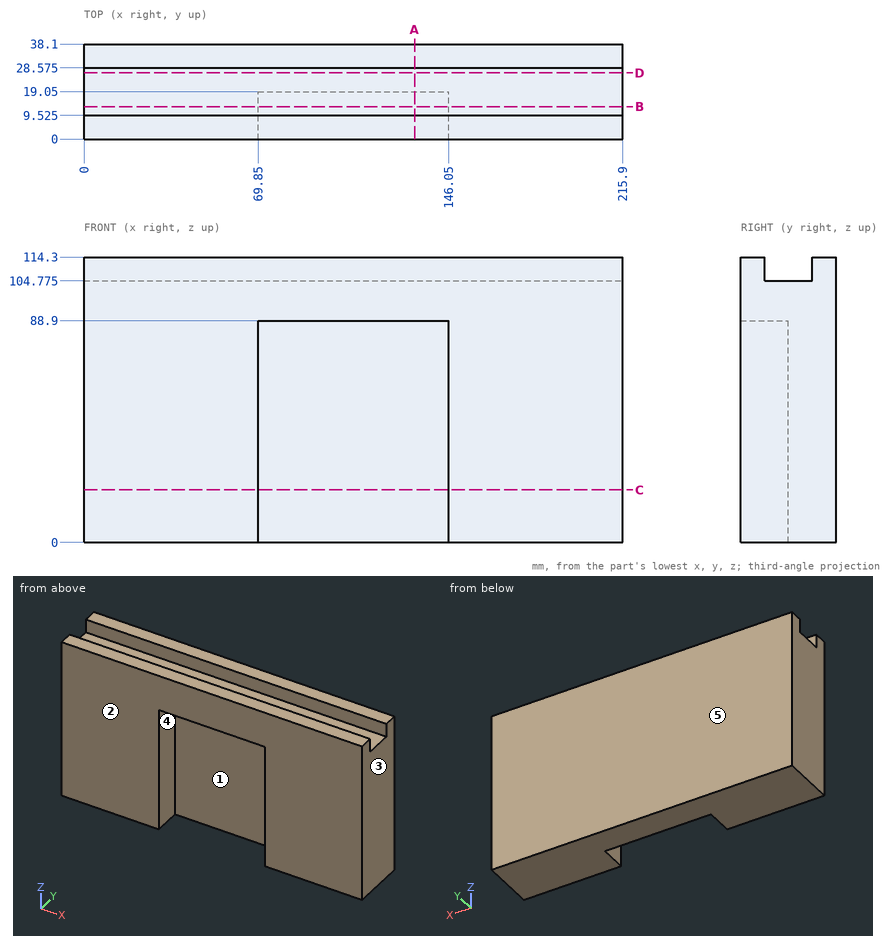
The figure shows three views and two pictorial views of one solid part (mm, origin at its lowest corner). Answer the questions. A direction names the side the tool comes from. Round coordinates to 2 decimals unless told otherwise and drop trailing zeros. Write each loop counter-clockwise with the first axis right and the second up, starting at its lowest first coordinate (ties: lowest second). Pieces come first, ordered by that corner, then holes. Notation, with made-up numbers: (-3.5, -30.5) - (31.5, -30.5) arc R36 cw to (31.5, 6.5) - close; hole circle Ø4 at (23.25, 17.25). An arc over 180 degrees is marked (long way). One line per question, with ' | ' between items. Start each with the question number.
1. For a pull along X with two mould halves and no side action, classify the marked faces 1, 2 and 3 as +X half, -X half, draft (parallel to the pull), parting line (faces both ways), or undercut.
2. Each of these flat-tipped pins is pushed along its axis until it touches: pin 1 (8 mm diameter, centred on x = 131.5, z = 82.5, fed in from -Y); pin 2 (9.5 mm diameter, centred on x = 91, y = 9, fed in from -Z); pin 3 (15 mm diameter, centred on x = 132, y = 21, fed in from +Z) (3 decimals). Where does it stop, or does it pass through?
3. Section B-B (y = 13) is taken. Determine the outline of the cut face in (x, z) (3 decimals), and give its area (3 significant figures).
4. Section D-D (y = 26.5) is taken. Determine the outline of the cut face in (x, z) (3 decimals).
5. Section A-A (x = 132.5) is taken. Determine the outline of the cut face in (y, z) (3 decimals).
6. For the marked faces 4 and 5, determine the directions among +Z, -Z, +X, -X, +Y, -Y from which every point of the face is accessible in a straight line to the end or side of a thin tool.
7. Section C-C (z = 21) is taken. Determine the outline of the cut face in (x, y), and give its area (3 significant figures).
8. Find the intervals of material crossed by probe 1 along Y at (x, z) = (24, 106) (3 decimals); probe 2 along X at (y, z) = (7, 67); probe 3 along Y at (x, z) = (137, 63.5), in increasing order. Write a range as [from, to].
Filled in:
1) face 1: undercut | face 2: draft | face 3: +X half
2) pin 1: y = 19.05 | pin 2: z = 88.9 | pin 3: z = 104.775
3) outline: (0, 0) - (69.85, 0) - (69.85, 88.9) - (146.05, 88.9) - (146.05, 0) - (215.9, 0) - (215.9, 104.775) - (0, 104.775) - close | area: 15,800 mm²
4) outline: (0, 0) - (215.9, 0) - (215.9, 104.775) - (0, 104.775) - close
5) outline: (0, 88.9) - (19.05, 88.9) - (19.05, 0) - (38.1, 0) - (38.1, 114.3) - (28.575, 114.3) - (28.575, 104.775) - (9.525, 104.775) - (9.525, 114.3) - (0, 114.3) - close
6) face 4: -Z, -Y | face 5: +Z, -Z, +X, -X, +Y
7) outline: (0, 0) - (69.85, 0) - (69.85, 19.05) - (146.05, 19.05) - (146.05, 0) - (215.9, 0) - (215.9, 38.1) - (0, 38.1) - close | area: 6,770 mm²
8) probe 1: [0, 9.525], [28.575, 38.1] | probe 2: [0, 69.85], [146.05, 215.9] | probe 3: [19.05, 38.1]
